Model file for the job. Use its own axes, mm. A direction names the side the tool comes from. Coordinates: 2 decimals unless noted, no trailing zeros. Order: outer loops, then holes, each group sorted by start corner. A loop starts at its lowest first (then second) coordinate and runs counter-clockwise, first axis right, second up.
from build123d import *

# Parameters (mm, degrees)
BOSS_EXTRUDE1_START        = -1.6
BOSS_EXTRUDE1_OUTLINE_W    = 25.3
BOSS_EXTRUDE1_OUTLINE_H    = 31.72
BOSS_EXTRUDE1_DEPTH        = 29.85
BOSS_EXTRUDE1_START_2      = 8
BOSS_EXTRUDE1_2_OUTLINE_W  = 25.3
BOSS_EXTRUDE1_2_OUTLINE_H  = 31.72
BOSS_EXTRUDE1_2_OUTLINE_R  = 5.125
BOSS_EXTRUDE1_2_DEPTH      = 12.25
BOSS_EXTRUDE1_3_OUTLINE_R  = 1.75
BOSS_EXTRUDE1_3_OUTLINE_W  = 25.3
BOSS_EXTRUDE1_3_OUTLINE_H  = 31.72
BOSS_EXTRUDE1_3_DEPTH      = 1.6
BOSS_EXTRUDE1_4_OUTLINE_R  = 5.125
BOSS_EXTRUDE1_4_OUTLINE_W  = 19.75
BOSS_EXTRUDE1_4_OUTLINE_H  = 8.3
BOSS_EXTRUDE1_4_DEPTH      = 16.14
BOSS_EXTRUDE1_5_OUTLINE_W  = 6.35
BOSS_EXTRUDE1_5_OUTLINE_H  = 12.7
BOSS_EXTRUDE1_5_DEPTH      = 9
BOSS_EXTRUDE1_START_3      = 28.25
BOSS_EXTRUDE1_6_DEPTH      = 1.75
BOSS_EXTRUDE1_7_OUTLINE_W  = 7.2
BOSS_EXTRUDE1_7_OUTLINE_H  = 7.2
BOSS_EXTRUDE1_7_DEPTH      = 4.5
BOSS_EXTRUDE1_START_4      = 16.14
BOSS_EXTRUDE1_8_OUTLINE_W  = 19.75
BOSS_EXTRUDE1_8_OUTLINE_H  = 8.3
BOSS_EXTRUDE1_8_DEPTH      = 0.61
BOSS_EXTRUDE1_START_5      = -1.5
BOSS_EXTRUDE1_9_OUTLINE_W  = 5.1
BOSS_EXTRUDE1_9_OUTLINE_H  = 1.7
BOSS_EXTRUDE1_9_DEPTH      = 1.5
BOSS_EXTRUDE1_START_6      = 20.25
BOSS_EXTRUDE1_10_OUTLINE_R = 5.125
BOSS_EXTRUDE1_10_DEPTH     = 0.39
CUT_EXTRUDE1_START         = -1.5
SKETCH1_3_W                = 125.683572393
SKETCH1_3_H                = 110.20529993
SKETCH1_3_W_2              = 88.9
SKETCH1_3_H_2              = 82.35
SKETCH1_3_R                = 1.75
SKETCH1_3_W_3              = 5.1
SKETCH1_3_H_3              = 2
CUT_EXTRUDE1_DEPTH         = 1.5
CHAMFER1_SIZE              = 2
SKETCH2_W                  = 2.7
SKETCH2_H                  = 4
BOSS_EXTRUDE2_DEPTH        = 4.4
SKETCH3_R                  = 0.5
BOSS_EXTRUDE3_DEPTH        = 3
MOVE_FACE1_BY              = 2.6
MOVE_FACE2_BY              = 0.36


with BuildPart() as part:
    # Boss-Extrude1: read off the stored shape, not the designer's step
    # Boss-Extrude1 outline → Boss-Extrude1 (new body)
    with BuildSketch(Plane(origin=(-2.49, 0, 0), x_dir=(0, 0, -1), z_dir=(1, 0, 0)).offset(BOSS_EXTRUDE1_START)):
        with Locations((-263.102543264, -6.78)):
            Rectangle(BOSS_EXTRUDE1_OUTLINE_W, BOSS_EXTRUDE1_OUTLINE_H)
        Polygon((-240.09, 28.14), (-245.61, 28.14), (-245.61, 36.25), (-246.67, 36.25), (-246.67, 28.14), (-251.07, 28.14), (-251.07, 36.25), (-252.13, 36.25), (-252.13, 28.14), (-259.98, 28.14), (-259.98, 36.25), (-261.04, 36.25), (-261.04, 30.75), (-262.415, 30.75), (-262.415, 28.75), (-263.915, 28.75), (-263.915, 30.75), (-265.29, 30.75), (-265.29, 36.25), (-266.35, 36.25), (-266.35, 19.25), (-265.1, 19.25), (-265.1, 26.14), (-220.6, 26.14), (-220.6, 19.25), (-219.35, 19.25), (-219.35, 36.25), (-220.41, 36.25), (-220.41, 30.75), (-221.785, 30.75), (-221.785, 28.75), (-223.285, 28.75), (-223.285, 30.75), (-224.66, 30.75), (-224.66, 36.25), (-225.72, 36.25), (-225.72, 28.14), (-233.57, 28.14), (-233.57, 36.25), (-234.63, 36.25), (-234.63, 28.14), (-239.03, 28.14), (-239.03, 36.25), (-240.09, 36.25), align=None)
    extrude(amount=BOSS_EXTRUDE1_DEPTH)

    # Boss-Extrude1 2 outline → Boss-Extrude1 2 (add)
    # profile 1 of 2: a face of its own
    with BuildSketch(Plane(origin=(-2.49, 0, 0), x_dir=(0, 0, -1), z_dir=(1, 0, 0)).offset(BOSS_EXTRUDE1_START_2)):
        with BuildLine():
            ThreePointArc((-280.252543264, 15.08), (-281.313203436, 14.640660172), (-281.752543264, 13.58))
            Line((-281.752543264, 13.58), (-281.752543264, -27.14))
            ThreePointArc((-281.752543264, -27.14), (-281.313203436, -28.200660172), (-280.252543264, -28.64))
            Line((-280.252543264, -28.64), (-245.952543264, -28.64))
            ThreePointArc((-245.952543264, -28.64), (-244.891883092, -28.200660172), (-244.452543264, -27.14))
            Line((-244.452543264, -27.14), (-244.452543264, 13.58))
            ThreePointArc((-244.452543264, 13.58), (-244.891883092, 14.640660172), (-245.952543264, 15.08))
            Line((-245.952543264, 15.08), (-280.252543264, 15.08))
        make_face()
        with Locations((-263.102543264, -6.78)):
            Rectangle(BOSS_EXTRUDE1_2_OUTLINE_W, BOSS_EXTRUDE1_2_OUTLINE_H, mode=Mode.SUBTRACT)
    # profile 2 of 2: a face of its own
    with BuildSketch(Plane(origin=(-2.49, 0, 0), x_dir=(0, 0, -1), z_dir=(1, 0, 0)).offset(BOSS_EXTRUDE1_START_2)):
        with Locations((-222.447456736, 11.25)):
            Circle(BOSS_EXTRUDE1_2_OUTLINE_R)
    extrude(amount=BOSS_EXTRUDE1_2_DEPTH)

    # Boss-Extrude1 3 outline → Boss-Extrude1 3 (add)
    with BuildSketch(Plane(origin=(-2.49, 0, 0), x_dir=(0, 0, -1), z_dir=(1, 0, 0)).offset(BOSS_EXTRUDE1_START)):
        Polygon((-251.4, -42.3), (-251.4, -44.3), (-234.3, -44.3), (-234.3, -42.3), (-229.2, -42.3), (-229.2, -44.3), (-198.4, -44.3), (-198.4, 38.05), (-287.3, 38.05), (-287.3, -44.3), (-256.5, -44.3), (-256.5, -42.3), align=None)
        with Locations((-282.3, -39.3)):
            Circle(BOSS_EXTRUDE1_3_OUTLINE_R, mode=Mode.SUBTRACT)
        with Locations((-203.4, -39.3)):
            Circle(BOSS_EXTRUDE1_3_OUTLINE_R, mode=Mode.SUBTRACT)
        with Locations((-282.3, 33.05)):
            Circle(BOSS_EXTRUDE1_3_OUTLINE_R, mode=Mode.SUBTRACT)
        Polygon((-245.61, 36.25), (-245.61, 28.14), (-240.09, 28.14), (-240.09, 36.25), (-239.03, 36.25), (-239.03, 28.14), (-234.63, 28.14), (-234.63, 36.25), (-233.57, 36.25), (-233.57, 28.14), (-225.72, 28.14), (-225.72, 36.25), (-224.66, 36.25), (-224.66, 30.75), (-223.285, 30.75), (-223.285, 28.75), (-221.785, 28.75), (-221.785, 30.75), (-220.41, 30.75), (-220.41, 36.25), (-219.35, 36.25), (-219.35, 19.25), (-220.6, 19.25), (-220.6, 26.14), (-265.1, 26.14), (-265.1, 19.25), (-266.35, 19.25), (-266.35, 36.25), (-265.29, 36.25), (-265.29, 30.75), (-263.915, 30.75), (-263.915, 28.75), (-262.415, 28.75), (-262.415, 30.75), (-261.04, 30.75), (-261.04, 36.25), (-259.98, 36.25), (-259.98, 28.14), (-252.13, 28.14), (-252.13, 36.25), (-251.07, 36.25), (-251.07, 28.14), (-246.67, 28.14), (-246.67, 36.25), align=None, mode=Mode.SUBTRACT)
        with Locations((-203.4, 33.05)):
            Circle(BOSS_EXTRUDE1_3_OUTLINE_R, mode=Mode.SUBTRACT)
        with Locations((-263.102543264, -6.78)):
            Rectangle(BOSS_EXTRUDE1_3_OUTLINE_W, BOSS_EXTRUDE1_3_OUTLINE_H, mode=Mode.SUBTRACT)
    extrude(amount=BOSS_EXTRUDE1_3_DEPTH)

    # Boss-Extrude1 4 outline → Boss-Extrude1 4 (add)
    with BuildSketch(Plane(origin=(-2.49, 0, 0), x_dir=(0, 0, -1), z_dir=(1, 0, 0))):
        with Locations((-221.216821393, -1.35)):
            Circle(BOSS_EXTRUDE1_4_OUTLINE_R)
        with Locations((-242.85, -37)):
            Rectangle(BOSS_EXTRUDE1_4_OUTLINE_W, BOSS_EXTRUDE1_4_OUTLINE_H)
        with Locations((-222.447456736, 11.25)):
            Circle(BOSS_EXTRUDE1_4_OUTLINE_R)
    extrude(amount=BOSS_EXTRUDE1_4_DEPTH)

    # Boss-Extrude1 5 outline → Boss-Extrude1 5 (add)
    with BuildSketch(Plane(origin=(-2.49, 0, 0), x_dir=(0, 0, -1), z_dir=(1, 0, 0))):
        with Locations((-202.972456736, 0)):
            Rectangle(BOSS_EXTRUDE1_5_OUTLINE_W, BOSS_EXTRUDE1_5_OUTLINE_H)
    extrude(amount=BOSS_EXTRUDE1_5_DEPTH)

    # Boss-Extrude1 6 outline → Boss-Extrude1 6 (add)
    with BuildSketch(Plane(origin=(-2.49, 0, 0), x_dir=(0, 0, -1), z_dir=(1, 0, 0)).offset(BOSS_EXTRUDE1_START_3)):
        Polygon((-240.09, 28.14), (-245.61, 28.14), (-245.61, 36.25), (-246.67, 36.25), (-246.67, 28.14), (-251.07, 28.14), (-251.07, 36.25), (-252.13, 36.25), (-252.13, 28.14), (-259.98, 28.14), (-259.98, 36.25), (-261.04, 36.25), (-261.04, 30.75), (-262.415, 30.75), (-262.415, 28.75), (-263.915, 28.75), (-263.915, 30.75), (-265.29, 30.75), (-265.29, 36.25), (-266.35, 36.25), (-266.35, 19.25), (-265.1, 19.25), (-265.1, 26.14), (-220.6, 26.14), (-220.6, 19.25), (-219.35, 19.25), (-219.35, 36.25), (-220.41, 36.25), (-220.41, 30.75), (-221.785, 30.75), (-221.785, 28.75), (-223.285, 28.75), (-223.285, 30.75), (-224.66, 30.75), (-224.66, 36.25), (-225.72, 36.25), (-225.72, 28.14), (-233.57, 28.14), (-233.57, 36.25), (-234.63, 36.25), (-234.63, 28.14), (-239.03, 28.14), (-239.03, 36.25), (-240.09, 36.25), align=None)
    extrude(amount=BOSS_EXTRUDE1_6_DEPTH)

    # Boss-Extrude1 7 outline → Boss-Extrude1 7 (add)
    with BuildSketch(Plane(origin=(-2.49, 0, 0), x_dir=(0, 0, -1), z_dir=(1, 0, 0))):
        with Locations((-232.947456736, -6)):
            Rectangle(BOSS_EXTRUDE1_7_OUTLINE_W, BOSS_EXTRUDE1_7_OUTLINE_H)
    extrude(amount=BOSS_EXTRUDE1_7_DEPTH)

    # Boss-Extrude1 8 outline → Boss-Extrude1 8 (add)
    with BuildSketch(Plane(origin=(-2.49, 0, 0), x_dir=(0, 0, -1), z_dir=(1, 0, 0)).offset(BOSS_EXTRUDE1_START_4)):
        with Locations((-242.85, -37)):
            Rectangle(BOSS_EXTRUDE1_8_OUTLINE_W, BOSS_EXTRUDE1_8_OUTLINE_H)
    extrude(amount=BOSS_EXTRUDE1_8_DEPTH)

    # Boss-Extrude1 9 outline → Boss-Extrude1 9 (add)
    with BuildSketch(Plane(origin=(-2.49, 0, 0), x_dir=(0, 0, -1), z_dir=(1, 0, 0)).offset(BOSS_EXTRUDE1_START_5)):
        with Locations((-253.95, -43.15)):
            Rectangle(BOSS_EXTRUDE1_9_OUTLINE_W, BOSS_EXTRUDE1_9_OUTLINE_H)
        with Locations((-231.75, -43.15)):
            Rectangle(BOSS_EXTRUDE1_9_OUTLINE_W, BOSS_EXTRUDE1_9_OUTLINE_H)
        Polygon((-287.752543264, -23.847456736), (-287.3, -24.3), (-287.3, 24.580582618), (-287.752543264, 24.580582618), align=None)
        Polygon((-198.4, 26.105086528), (-198.4, -24.3), (-197.947456736, -23.847456736), (-197.947456736, 25.652543264), align=None)
        with BuildLine():
            Line((-281.502543264, 33.330582618), (-281.502543264, 31.492257161))
            ThreePointArc((-281.502543264, 31.492257161), (-280.609414894, 32.597869487), (-280.831414071, 34.00171181))
            Line((-280.831414071, 34.00171181), (-281.502543264, 33.330582618))
        make_face()
        with BuildLine():
            Line((-203.60722612, 31.312312647), (-205.137687353, 32.84277388))
            ThreePointArc((-205.137687353, 32.84277388), (-204.637436867, 31.812563133), (-203.60722612, 31.312312647))
        make_face()
    extrude(amount=BOSS_EXTRUDE1_9_DEPTH)

    # Boss-Extrude1 10 outline → Boss-Extrude1 10 (add)
    with BuildSketch(Plane(origin=(-2.49, 0, 0), x_dir=(0, 0, -1), z_dir=(1, 0, 0)).offset(BOSS_EXTRUDE1_START_6)):
        with Locations((-222.447456736, 11.25)):
            Circle(BOSS_EXTRUDE1_10_OUTLINE_R)
    extrude(amount=BOSS_EXTRUDE1_10_DEPTH)

    # Sketch1<3> → Cut-Extrude1 (cut)
    # profile 1 of 7: a face of its own
    with BuildSketch(Plane(origin=(-2.49, 0, 0), x_dir=(0, 0, -1), z_dir=(1, 0, 0)).offset(CUT_EXTRUDE1_START)):
        with Locations((-237.633848224, 0.203353058)):
            Rectangle(SKETCH1_3_W, SKETCH1_3_H)
        with Locations((-242.85, -3.125)):
            Rectangle(SKETCH1_3_W_2, SKETCH1_3_H_2, mode=Mode.SUBTRACT)
    # profile 2 of 7: a face of its own
    with BuildSketch(Plane(origin=(-2.49, 0, 0), x_dir=(0, 0, -1), z_dir=(1, 0, 0)).offset(CUT_EXTRUDE1_START)):
        with Locations((-282.3, 33.05)):
            Circle(SKETCH1_3_R)
    # profile 3 of 7: a face of its own
    with BuildSketch(Plane(origin=(-2.49, 0, 0), x_dir=(0, 0, -1), z_dir=(1, 0, 0)).offset(CUT_EXTRUDE1_START)):
        with Locations((-203.4, 33.05)):
            Circle(SKETCH1_3_R)
    # profile 4 of 7: a face of its own
    with BuildSketch(Plane(origin=(-2.49, 0, 0), x_dir=(0, 0, -1), z_dir=(1, 0, 0)).offset(CUT_EXTRUDE1_START)):
        with Locations((-203.4, -39.3)):
            Circle(SKETCH1_3_R)
    # profile 5 of 7: a face of its own
    with BuildSketch(Plane(origin=(-2.49, 0, 0), x_dir=(0, 0, -1), z_dir=(1, 0, 0)).offset(CUT_EXTRUDE1_START)):
        with Locations((-282.3, -39.3)):
            Circle(SKETCH1_3_R)
    # profile 6 of 7: a face of its own
    with BuildSketch(Plane(origin=(-2.49, 0, 0), x_dir=(0, 0, -1), z_dir=(1, 0, 0)).offset(CUT_EXTRUDE1_START)):
        with Locations((-253.95, -43.3)):
            Rectangle(SKETCH1_3_W_3, SKETCH1_3_H_3)
    # profile 7 of 7: a face of its own
    with BuildSketch(Plane(origin=(-2.49, 0, 0), x_dir=(0, 0, -1), z_dir=(1, 0, 0)).offset(CUT_EXTRUDE1_START)):
        with Locations((-231.75, -43.3)):
            Rectangle(SKETCH1_3_W_3, SKETCH1_3_H_3)
    extrude(amount=CUT_EXTRUDE1_DEPTH, mode=Mode.SUBTRACT)

    # Chamfer1
    chamfer1_edges = [part.edges().sort_by_distance(p)[0] for p in [
        (-3.29, -44.3, 287.3),
        (-3.29, 38.05, 198.4),
        (-3.29, 38.05, 287.3),
        (-3.29, -44.3, 198.4),
    ]]
    chamfer(chamfer1_edges, length=CHAMFER1_SIZE)

    # Sketch2 → Boss-Extrude2 (add)
    with BuildSketch(Plane(origin=(-2.49, 0, 0), x_dir=(0, 0, -1), z_dir=(1, 0, 0))):
        with Locations((-273.15, 30.62)):
            Rectangle(SKETCH2_W, SKETCH2_H)
    extrude(amount=BOSS_EXTRUDE2_DEPTH)

    # Sketch3 → Boss-Extrude3 (add)
    with BuildSketch(Plane.ZY.offset(4.09)):
        with Locations(Location((234.85, -37.3, 0), (0, 0, 180))):
            Circle(SKETCH3_R)
        with Locations(Location((250.85, -37.3, 0), (0, 0, 180))):
            Circle(SKETCH3_R)
    extrude(amount=BOSS_EXTRUDE3_DEPTH)

    # Move Face1: a face moved outward by 2.6
    extrude(part.faces().sort_by_distance((27.51, 27.75, 242.85))[0], amount=MOVE_FACE1_BY, dir=(1, 0, 0))

    # Move Face2: a face moved outward by 0.36
    extrude(part.faces().sort_by_distance((13.65, -1.35, 221.216821393))[0], amount=MOVE_FACE2_BY, dir=(1, 0, 0))


solid = part.part
Q1. Probe line 1 (Y direction, x = -3.1, z = 282.3); line 2 (Z direction, x = 10.5, y = 22.5); line 3 (Y direction, x = 3, z = 223). List the from-to ranges inside material, lowest first.
Established:
line 1: y = -44.3 to -41.05, -37.55 to 31.3, 34.8 to 38.05
line 2: z = 219.35 to 220.6, 265.1 to 266.35
line 3: y = -6.15 to 3.45, 6.15 to 16.35, 26.14 to 28.75
Q2. Drop flat-ended pins along their axis: P1, Ø4.5, axis at x = 0, y = 31, coming from the -Z side; P2, Ø5, axis at x = 14, z = 252, coming from the -Y side; P3, Ø2.5, axis at x = 0, z = 263.5, coming from the -Y side. Give the stop position or say it passes through.
Established:
P1: stops at z = 219.35
P2: stops at y = -41.15
P3: stops at y = -22.64
Q3. Which spindle directions (+Z, -Z, +X, -X, +Y, -Y) get a long thin tool onto all of the face, cutting with end or side? Do faces 1 (the face through (1.91, 31, 273)), 2 (the face through (1, 9.08, 263)), 3 (the face through (14, 32, 240.09)). Say none if no direction does.
Established:
face 1: +Z, +X, +Y
face 2: +Z
face 3: +X, +Y
Q4. Cut at D-D, the plane y = 11.25. List the corners of the cut face in (x, z), plus the area to 3 significant figures.
Established:
outline: (-4.09, 198.4) - (-2.49, 198.4) - (-2.49, 217.32) - (18.15, 217.32) - (18.15, 227.57) - (-2.49, 227.57) - (-2.49, 287.3) - (-4.09, 287.3) - close; (5.51, 244.45) - (17.76, 244.45) - (17.76, 281.75) - (5.51, 281.75) - close
area: 811 mm2
Q5. Cut at B-B, the plane z = 203.4. List the corners of the cut face in (x, y), plus the area to 3 significant figures.
Established:
outline: (-4.09, -44.3) - (-2.49, -44.3) - (-2.49, -41.05) - (-4.09, -41.05) - close; (-4.09, -37.55) - (-2.49, -37.55) - (-2.49, -6.35) - (6.51, -6.35) - (6.51, 6.35) - (-2.49, 6.35) - (-2.49, 31.3) - (-4.09, 31.3) - close; (-4.09, 34.8) - (-2.49, 34.8) - (-2.49, 38.05) - (-4.09, 38.05) - close
area: 235 mm2
Q6. Mould opens along Y. For faces 4 (the face through (5.51, -6, 276)), 5 (the face through (-3.28, 37.04, 199.39)), 6 (the face through (0, 31, 271.8)) say: pulls with the +Y half, pulls with the -Y half, needs draft (parallel to the pull), parting line crosses it, or undercut.
Established:
face 4: undercut
face 5: pulls with the +Y half
face 6: needs draft
Q7. Cut at A-A, the plane y = -24.5. List the corners of the cut face in (x, z).
Established:
outline: (-4.09, 198.4) - (-2.49, 198.4) - (-2.49, 287.3) - (-4.09, 287.3) - close; (5.51, 244.45) - (17.76, 244.45) - (17.76, 281.75) - (5.51, 281.75) - close
Q8. Cut at C-C, the plane y = 24.5. List the corners of the cut face in (x, z).
Established:
outline: (-4.09, 198.4) - (-2.49, 198.4) - (-2.49, 219.35) - (30.11, 219.35) - (30.11, 220.6) - (-2.49, 220.6) - (-2.49, 265.1) - (30.11, 265.1) - (30.11, 266.35) - (-2.49, 266.35) - (-2.49, 287.3) - (-4.09, 287.3) - close
